Could you check a few things on this model? Use its own coordinates, in mm. A direction names the side the tool comes from. Coordinates: 2 decimals unless noted, no trailing zeros. Order: outer loops, then holes, each group sorted by start corner. A loop starts at its lowest first (then second) coordinate and runs counter-clockwise, first axis right, second up. Notation, with made-up numbers: (-34, 10) -> (-1, 10) arc R11 ccw to (-1, 28) -> close; hole circle Ø2 at (23, -39). An arc over 180 degrees is marked (long way). Put each result on its own line as item: value. Start each with the question number.
Q1. If we section it at C-C (y = 170): Please give me the cut outline in (x, z).
Q2. We'd pull the mould along X, two halves only. Please class faces 1 (the face through (213.251, 168, 1)), 2 (the face through (207.645, 162.442, 1.479)), 3 (the face through (217.556, 162.916, 1.479)), 4 (the face through (209, 159, 0)): +X half, -X half, draft (parallel to the pull), parting line (faces both ways), or undercut.
Q3. Please list where these lines run through material, in increasing order: line 1 along X through (y, z) = (167.5, 0.15); line 2 along X through (y, z) = (160.5, 0.55); line 3 along X through (y, z) = (170.25, 2).
Q4. Will these pins go through, and if not, where does the flat tip stop? pin 1 (0.9 mm diameter, centred on x = 215, z = 1, fed in from +Y); pin 2 (1.5 mm diameter, centred on y = 170, z = 2.5, fed in from +X); pin 3 (0.9 mm diameter, centred on y = 155.5, z = 2, fed in from -X).
Q5. For faces 5 (the face through (215, 156.928, 1)), 6 (the face through (216, 165.928, 1)), 7 (the face through (202, 156.928, 1)), 8 (the face through (202, 165.928, 1)), which set-ups out of +Z, -Z, +X, -X, +Y, -Y let a thin tool reach every point of the face, with its end or its side?
Q6. If we section it at D-D (z = 1.8): Please give me the cut outline in (x, y).
Q7. If we section it at A-A (y = 162.25): Please give me the cut outline in (x, z).
Q8. If we section it at B-B (x = 199.25): Please give me the cut outline in (y, z), and give its area (3 significant figures).
from build123d import *

# Parameters (mm, degrees)
MODEL_R                 = 1.5
SALIENTE_EXTRUIR1_DEPTH = 3


with BuildPart() as part:
    # Model → Saliente-Extruir1 (new body)
    with BuildSketch(Plane.XY):
        with BuildLine():
            Line((213.25077615, 165.928489513), (213.25077615, 170.428489513))
            ThreePointArc((213.25077615, 170.428489513), (208.75077615, 174.928489513), (204.25077615, 170.428489513))
            Line((204.25077615, 170.428489513), (204.25077615, 165.928489513))
            Line((204.25077615, 165.928489513), (199.75077615, 165.928489513))
            ThreePointArc((199.75077615, 165.928489513), (195.25077615, 161.428489513), (199.75077615, 156.928489513))
            Line((199.75077615, 156.928489513), (204.25077615, 156.928489513))
            Line((204.25077615, 156.928489513), (204.25077615, 152.428489513))
            ThreePointArc((204.25077615, 152.428489513), (208.75077615, 147.928489513), (213.25077615, 152.428489513))
            Line((213.25077615, 152.428489513), (213.25077615, 156.928489513))
            Line((213.25077615, 156.928489513), (217.75077615, 156.928489513))
            ThreePointArc((217.75077615, 156.928489513), (222.25077615, 161.428489513), (217.75077615, 165.928489513))
            Line((217.75077615, 165.928489513), (213.25077615, 165.928489513))
        make_face()
        with Locations((208.75077615, 152.428489513)):
            Circle(MODEL_R, mode=Mode.SUBTRACT)
        with Locations((208.75077615, 161.428489513)):
            Circle(MODEL_R, mode=Mode.SUBTRACT)
        with Locations((208.75077615, 170.428489513)):
            Circle(MODEL_R, mode=Mode.SUBTRACT)
        with Locations((199.75077615, 161.428489513)):
            Circle(MODEL_R, mode=Mode.SUBTRACT)
        with Locations((217.75077615, 161.428489513)):
            Circle(MODEL_R, mode=Mode.SUBTRACT)
    extrude(amount=SALIENTE_EXTRUIR1_DEPTH)


solid = part.part
The answers:
1. outline: (204.25, 0) -> (207.31, 0) -> (207.31, 3) -> (204.25, 3) -> close; (210.19, 0) -> (213.25, 0) -> (213.25, 3) -> (210.19, 3) -> close
2. face 1: +X half
2. face 2: undercut
2. face 3: undercut
2. face 4: draft
3. line 1: 204.25 to 213.25
3. line 2: 195.35 to 198.57, 200.93 to 207.57, 209.93 to 216.57, 218.93 to 222.15
3. line 3: 204.25 to 207.26, 210.24 to 213.25
4. pin 1: y = 165.93
4. pin 2: x = 213.25
4. pin 3: x = 204.25
5. face 5: +Z, -Z, +X, -Y
5. face 6: +Z, -Z, +X, +Y
5. face 7: +Z, -Z, -X, -Y
5. face 8: +Z, -Z, -X, +Y
6. outline: (199.75, 156.93) -> (204.25, 156.93) -> (204.25, 152.43) arc R4.5 ccw to (213.25, 152.43) -> (213.25, 156.93) -> (217.75, 156.93) arc R4.5 ccw to (217.75, 165.93) -> (213.25, 165.93) -> (213.25, 170.43) arc R4.5 ccw to (204.25, 170.43) -> (204.25, 165.93) -> (199.75, 165.93) arc R4.5 ccw to start; hole circle Ø3 at (199.75, 161.43); hole circle Ø3 at (208.75, 152.43); hole circle Ø3 at (208.75, 161.43); hole circle Ø3 at (208.75, 170.43); hole circle Ø3 at (217.75, 161.43)
7. outline: (195.33, 0) -> (198.5, 0) -> (198.5, 3) -> (195.33, 3) -> close; (201.01, 0) -> (207.5, 0) -> (207.5, 3) -> (201.01, 3) -> close; (210.01, 0) -> (216.5, 0) -> (216.5, 3) -> (210.01, 3) -> close; (219.01, 0) -> (222.18, 0) -> (222.18, 3) -> (219.01, 3) -> close
8. outline: (156.96, 0) -> (160.01, 0) -> (160.01, 3) -> (156.96, 3) -> close; (162.84, 0) -> (165.9, 0) -> (165.9, 3) -> (162.84, 3) -> close
8. area: 18.3 mm^2
